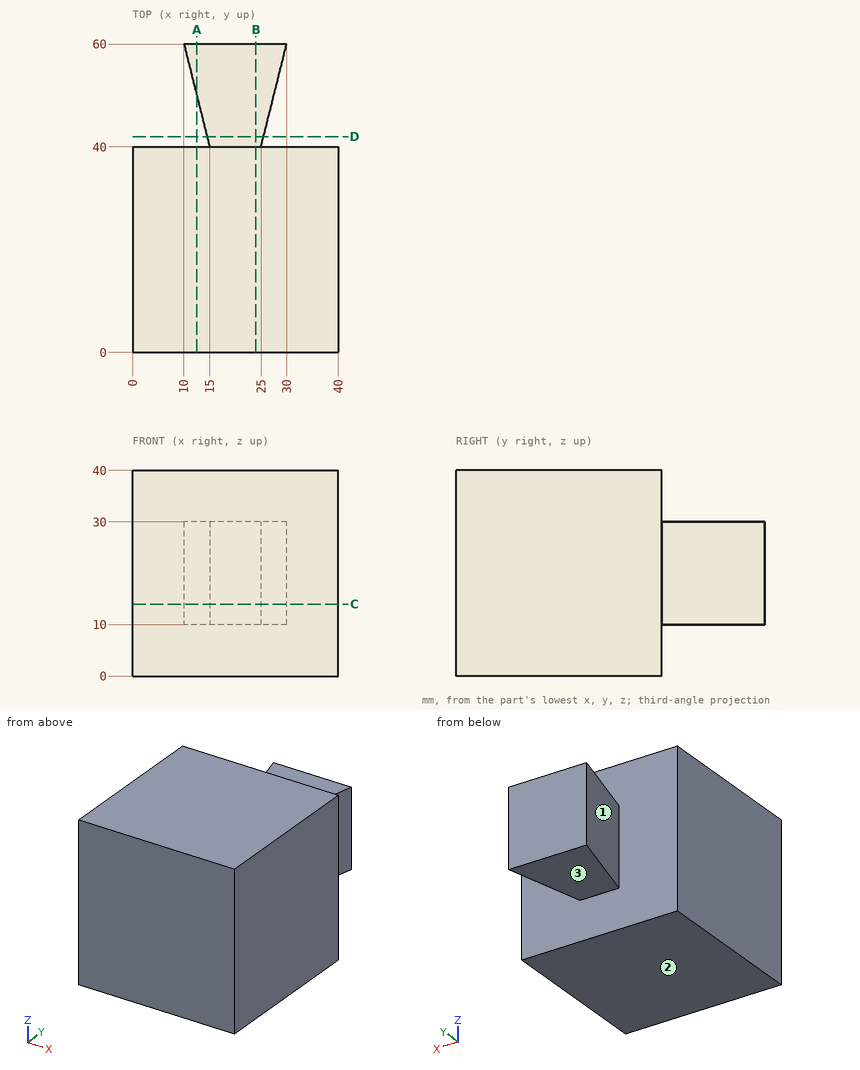
Geometry: see drawing. Coordinates: mm, zero at the bounding-box minimum. A direction names the side the tool comes from. Give positions to 0.01 mm unless a question says otherwise; leave off trailing zeros. Loops run counter-clockwise (first coordinate to the right, second up) from the corner with the lowest first, then second, coordinate; pieces in that order, holes last. Notation, with made-up numbers: (86, 1) - (106, 1) arc R7 ccw to (106, 10) - close; hole circle Ø2 at (-7.75, -36). An arc over 180 degrees is marked (long way). Answer as CSV lines item,"result". Start each with the question number.
1. Section C-C, the plane z = 14. Return loops of the section in (x, y), plus the area to 3 significant figures.
2. Pin query (flat end, axial travel): P1, Ø4, axis at x = 15.5, y = 48, coming from the +Z side; P2, Ø8, axis at x = 34, y = 54, coming from the -Z side; P3, Ø1.5, axis at y = 37, z = 21, coming from the -X side; P4, Ø16, axis at x = 21, y = 51, coming from the -Z side. Return the tip coordinate at first contact, or that it passes through.
3. Section D-D, the plane y = 42. Return loops of the section in (x, z).
4. Section A-A, the plane x = 12.5. Return loops of the section in (y, z).
5. Reachability of the marked faces 1, 2 and 3 from +Z, -Z, +X, -X, +Y, -Y: full face, straight path, thin tool, end or side. Return the list, or none.
6. Section B-B, the plane x = 24. Return loops of the section in (y, z), plus the area to 3 significant figures.
7. Ray query, L1, parallel to Y at x = 26, z = 4; L2, parallel to Z at x = 16, y = 51.5; L3, parallel to X at y = 42, z = 24. Return the intervals inside material, ascending.
Answers:
1,outline,"(0, 0) - (40, 0) - (40, 40) - (25, 40) - (30, 60) - (10, 60) - (15, 40) - (0, 40) - close"
1,area,"1,900 mm2"
2,P1,"stops at z = 30"
2,P2,"passes through"
2,P3,"stops at x = 0"
2,P4,"stops at z = 10"
3,outline,"(14.5, 10) - (25.5, 10) - (25.5, 30) - (14.5, 30) - close"
4,outline,"(0, 0) - (40, 0) - (40, 40) - (0, 40) - close; (50, 10) - (60, 10) - (60, 30) - (50, 30) - close"
5,face 1,"+Z, -Z, -X"
5,face 2,"-Z, +X, -X, +Y, -Y"
5,face 3,"-Z, +X, -X, +Y"
6,outline,"(0, 0) - (40, 0) - (40, 10) - (60, 10) - (60, 30) - (40, 30) - (40, 40) - (0, 40) - close"
6,area,"2,000 mm2"
7,L1,"y = 0 to 40"
7,L2,"z = 10 to 30"
7,L3,"x = 14.5 to 25.5"
